from build123d import *

# Parameters (mm, degrees)
SKETCH_W     = 53
SKETCH_H     = 22.5
PAD_DEPTH    = 4
SKETCH001_W  = 50
SKETCH001_H  = 20
POCKET_DEPTH = 3.5
SKETCH002_W  = 2.5
SKETCH002_H  = 2.5
PAD001_DEPTH = 4


with BuildPart() as part:
    # Sketch → Pad (new body)
    with BuildSketch(Plane.XY):
        Rectangle(SKETCH_W, SKETCH_H)
    extrude(amount=PAD_DEPTH)

    # Sketch001 (on Face6 of Pad) → Pocket (cut)
    with BuildSketch(Plane.XY.offset(4)):
        with Locations((0, 1.25)):
            Rectangle(SKETCH001_W, SKETCH001_H)
    extrude(amount=-POCKET_DEPTH, mode=Mode.SUBTRACT)

    # Sketch002 (on Face4 of Pocket) → Pad001 (join)
    with BuildSketch(Plane.XY.offset(4)):
        with Locations((-18, -10)):
            Rectangle(SKETCH002_W, SKETCH002_H)
        with Locations((-13, -10)):
            Rectangle(SKETCH002_W, SKETCH002_H)
        with Locations((-8, -10)):
            Rectangle(SKETCH002_W, SKETCH002_H)
    extrude(amount=PAD001_DEPTH)


with BuildPart() as part_1:
    # Body placement: moved
    add(part.part.moved(Location((0, -10, 0))))


solid = part_1.part
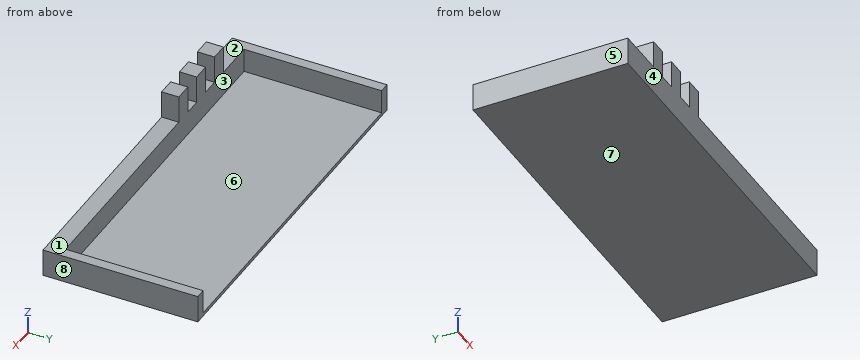
Could you check a few things on this model? Use its own coordinates, in mm. Face numbers are marked on the shaded views. A direction names the side the tool comes from. Give positions to 0.01 mm unless a question says otherwise; leave off trailing zeros. Loops run counter-clockwise (first coordinate to the right, second up) from the corner with the lowest first, then second, coordinate; pieces in that order, holes last. Notation, with made-up numbers: (60.25, 32.25) -> (65.25, 32.25) arc R21 cw to (65.25, 68.25) -> close; hole circle Ø6 at (21.5, 50.5). An arc over 180 degrees is marked (long way). Return JSON: item names as keys, results as strings.
Item 1: If we section it at A-A on z = 5: List the corners of the cut face in (x, y) for me.
Geometry results:
{"outline": "(-19.25, -21.25) -> (-16.75, -21.25) -> (-16.75, -18.75) -> (-19.25, -18.75) -> close; (-14.25, -21.25) -> (-11.75, -21.25) -> (-11.75, -18.75) -> (-14.25, -18.75) -> close; (-9.25, -21.25) -> (-6.75, -21.25) -> (-6.75, -18.75) -> (-9.25, -18.75) -> close"}
Item 2: I need wall thicknesses on L1, parallel to X at y = -19.75, z = 5.75; L2, parallel to X at y = -4.5, z = 1.75; L3, parallel to Y at x = 11.5, z = 3.75. Which ranges of each line are inside material? Lowest first, please. Write a range as from..to.
Geometry results:
{"L1": "x = -19.25..-16.75, -14.25..-11.75, -9.25..-6.75", "L2": "x = -26.5..-25, 25..26.5", "L3": "y = -21.25..-18.75"}
Item 3: If we section it at B-B on y = -2: List the corners of the cut face in (x, z) for me.
Geometry results:
{"outline": "(-26.5, 0) -> (26.5, 0) -> (26.5, 4) -> (25, 4) -> (25, 0.5) -> (-25, 0.5) -> (-25, 4) -> (-26.5, 4) -> close"}
Item 4: We'd pull the mould along X, two halves only. Please class the marked faces 6, 7 and 8: +X half, -X half, draft (parallel to the pull), parting line (faces both ways), or undercut.
Geometry results:
{"face 6": "undercut", "face 7": "draft", "face 8": "+X half"}
Item 5: If we section it at D-D on x = -13.5: List the corners of the cut face in (y, z) for me.
Geometry results:
{"outline": "(-21.25, 0) -> (1.25, 0) -> (1.25, 0.5) -> (-18.75, 0.5) -> (-18.75, 8) -> (-21.25, 8) -> close"}
Item 6: I'm going to push flat-ended pins straight in: pin 1 (0.8 mm diameter, centred on y = -19.5, z = 6.5, fed in from +X); pin 2 (8 mm diameter, centred on x = 14, y = -14, fed in from +Z); pin 3 (1.2 mm diameter, centred on x = -15, y = -19.5, fed in from +Z). Where does each tip first touch, or does it pass through?
Geometry results:
{"pin 1": "stops at x = -6.75", "pin 2": "stops at z = 0.5", "pin 3": "stops at z = 4"}
Item 7: If we section it at C-C on z = 1.75: List the corners of the cut face in (x, y) for me, plus the area to 4 significant figures.
Geometry results:
{"outline": "(-26.5, -21.25) -> (26.5, -21.25) -> (26.5, 1.25) -> (25, 1.25) -> (25, -18.75) -> (-25, -18.75) -> (-25, 1.25) -> (-26.5, 1.25) -> close", "area": "192.5 mm²"}
Item 8: Which directions (+Z, -Z, +X, -X, +Y, -Y) give clear straight access to the entire face, cutting with the end or side of a thin tool? Please do the marked faces 1, 2, 3, 4 and 5.
Geometry results:
{"face 1": "+Z, +X, +Y, -Y", "face 2": "+Z, -X, +Y, -Y", "face 3": "+Z, +Y", "face 4": "+Z, -Z, +X, -X, -Y", "face 5": "+Z, -Z, -X, +Y, -Y"}
